Geometry: final body of the model. Coordinates: model frame, mm. Round coordinates to 2 decimals unless told otherwise and drop trailing zeros. Loops run counter-clockwise (first coordinate to the right, second up) from the corner with the lowest first, then second, coordinate; pieces in that order, holes last. Notation, with made-up numbers: (-20.5, 34.5) - (17.5, 34.5) arc R13 ccw to (17.5, 59.5) - close; hole circle Ø10 at (78.5, 23.25). An arc over 180 degrees is marked (long way). Return JSON: item names as keys, results as strings. Group by question number.
1. Material intervals for probe 1 along Y at (x, z) = (7, -144.5); probe 2 along Z at (x, y) = (9.5, 63); probe 3 along Z at (x, y) = (1.75, 67.5), sorted ascending.
2. Section C-C on z = -86. Return loops of the section in (x, y), and give its area (3 significant figures).
3. Section B-B on x = 7.25. Return loops of the section in (y, z).
4. First-contact query: pin 1 Ø5 at (x, y) = (7, 66.5) entering from -Z. Flat tip, straight axial feed; report the tip coordinate or a pass-through.
5. Section A-A on y = 69. Return loops of the section in (x, z).
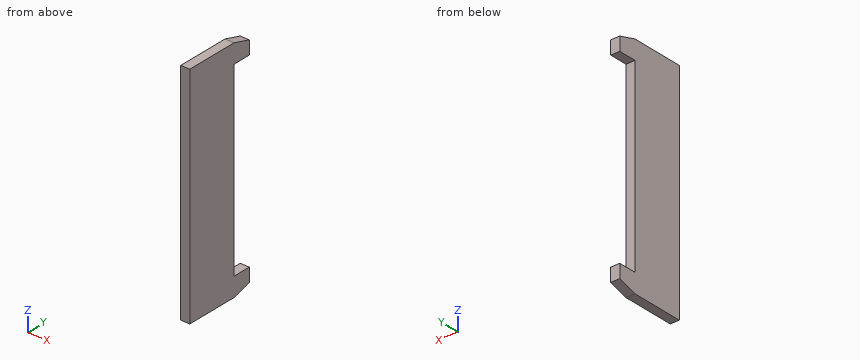
Autodesk Inventor part; units mm, degrees
ref_plane "YZ Plane" through (0, 0, 0) normal (1, 0, 0) x (0, 1, 0)
ref_plane "XZ Plane" through (0, 0, 0) normal (0, 1, 0) x (-1, 0, 0)
ref_plane "XY Plane" through (0, 0, 0) normal (0, 0, 1) x (1, 0, 0)
sketch "Sketch1" plane through (0, 0, 0) normal (1, 0, 0) x (0, 1, 0)
  line L0 (0, 0) -> (58, 0)
  line L1 (58, -250) -> (0, -250)
  line L2 (78, -6) -> (78, -21)
  line L3 (78, -21) -> (58, -21)
  line L4 (58, -21) -> (58, -125)
  line L5 (78, -21) -> (78, -6)
  line L6 (78, -21) -> (78, -6)
  line L7 (58, -229) -> (58, -125)
  line L8 (78, -229) -> (58, -229)
  line L9 (78, -244) -> (58, -250)
  line L10 (78, -244) -> (78, -229)
  line L11 (0, 0) -> (0, -62)
  line L12 (78, -6) -> (78, -21)
  line L13 (78, -229) -> (78, -244)
  line L14 (0, -250) -> (0, -75)
  line L15 (0, -62) -> (0, 0)
  line L16 (58, 0) -> (0, 0)
  line L17 (0, 0) -> (0, -62)
  line L18 (0, -75) -> (0, -250)
  line L19 (0, -250) -> (58, -250)
  line L20 (58, 0) -> (0, 0)
  line L21 (0, -62) -> (0, -75)
  line L22 (78, -6) -> (58, 0)
  dimension "d0" = 62
  dimension "d4" = 15
  dimension "d5" = 15
  dimension "d6" = 208
extrude "Extrusion1" add sketch "Sketch1" along normal blind 10
properties part number "Left Side" material "Steel"
Taken from the geometry:
{
 "1": {"probe 1": "0 to 58", "probe 2": "-248.5 to -229, -21 to -1.5", "probe 3": "-247.15 to -229, -21 to -2.85"},
 "2": {"outline": "(0, 0) - (10, 0) - (10, 58) - (0, 58) - close", "area": "580 mm2"},
 "3": {"outline": "(0, -250) - (58, -250) - (78, -244) - (78, -229) - (58, -229) - (58, -21) - (78, -21) - (78, -6) - (58, 0) - (0, 0) - close"},
 "4": {"pin 1": "z = -248.2"},
 "5": {"outline": "(0, -246.7) - (10, -246.7) - (10, -229) - (0, -229) - close; (0, -21) - (10, -21) - (10, -3.3) - (0, -3.3) - close"}
}
